from build123d import *

# Parameters (mm, degrees)
SKETCH1_R           = 2.5527
BOSS_EXTRUDE1_DEPTH = 127
SKETCH2_OUTSIDE_W   = 67.612
SKETCH2_OUTSIDE_H   = 65.648
SKETCH2_OUTSIDE_R   = 6.875
CUT_EXTRUDE1_DEPTH  = 25.4
SKETCH3_OUTSIDE_W   = 67.612
SKETCH3_OUTSIDE_H   = 65.648
SKETCH3_OUTSIDE_R   = 6.875
CUT_EXTRUDE2_DEPTH  = 12.7


with BuildPart() as part:
    # Sketch1 → Boss-Extrude1 (new, symmetric)
    with BuildSketch(Plane(origin=(0, 0, 0), x_dir=(0, 0, -1), z_dir=(1, 0, 0))):
        Polygon((3.666174209, -6.35), (7.332348419, 0), (3.666174209, 6.35), (-3.666174209, 6.35), (-7.332348419, 0), (-3.666174209, -6.35), align=None)
        Circle(SKETCH1_R, mode=Mode.SUBTRACT)
    extrude(amount=BOSS_EXTRUDE1_DEPTH, both=True)

    # Sketch2 outside → Cut-Extrude1 (cut)
    with BuildSketch(Plane.ZY.offset(127)):
        Rectangle(SKETCH2_OUTSIDE_W, SKETCH2_OUTSIDE_H)
        Circle(SKETCH2_OUTSIDE_R, mode=Mode.SUBTRACT)
    extrude(amount=-CUT_EXTRUDE1_DEPTH, mode=Mode.SUBTRACT)

    # Sketch3 outside → Cut-Extrude2 (cut)
    with BuildSketch(Plane(origin=(127, 0, 0), x_dir=(0, 0, -1), z_dir=(1, 0, 0))):
        Rectangle(SKETCH3_OUTSIDE_W, SKETCH3_OUTSIDE_H)
        Circle(SKETCH3_OUTSIDE_R, mode=Mode.SUBTRACT)
    extrude(amount=-CUT_EXTRUDE2_DEPTH, mode=Mode.SUBTRACT)


solid = part.part
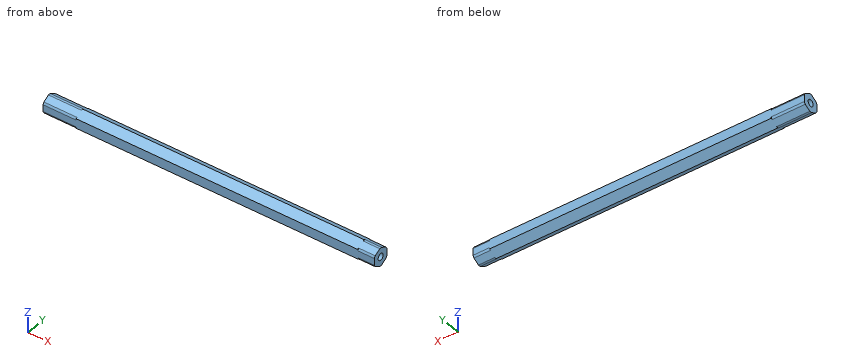
Build history of the part. All positions in model axes, mm. Round coordinates to 2 decimals unless told otherwise and drop trailing zeros. Write each loop counter-clockwise with the first axis right and the second up, starting at its lowest first coordinate (ties: lowest second). Pieces come first, ordered by that corner, then holes. Notation, with made-up numbers: M -3.75,6.5 L 11.25,6.5 A18 ccw 11.25,40.5 Z; hole C -13,-17 d1. An arc over 180 degrees is marked long. Answer as a JSON object with one key per item and string values. Group by question number.
(1) Drill centre lines: L1, parallel to Y at x = 0.5, z = 0.25; L2, parallel to Y at x = 74, z = 0; L3, parallel to Z at x = -50, y = 1.25. Where is each one in solid material? Low to high.
(2) Flat gauge pins, fed straight in: pin 1 (4 mm diameter, centred on y = 0, z = 0, fed in from +X); pin 2 (2 mm diameter, centred on x = 41, y = 3, fed in from +Z). Where does each tip first touch, or does it go through?
(3) Cut at A-A (z = 0). Give the cut face in (x, y).
(4) Cut at B-B (x = -75). Give the cut face in (y, z), and give its area (3 significant figures).
Responses:
{
 "1": {"L1": "y = -6.35 to -2.54, 2.54 to 6.35", "L2": "y = -6.35 to -2.55, 2.55 to 6.35", "L3": "z = -6.61 to -2.23, 2.23 to 6.61"},
 "2": {"pin 1": "passes through", "pin 2": "stops at z = 6.18"},
 "3": {"outline": "M -127,-6.35 L 127,-6.35 L 127,-2.55 L -127,-2.55 Z; M -127,2.55 L 127,2.55 L 127,6.35 L -127,6.35 Z"},
 "4": {"outline": "M -6.35,-3.67 L 0,-7.33 L 6.35,-3.67 L 6.35,3.67 L 0,7.33 L -6.35,3.67 Z; hole C 0,0 d5.11", "area": "119 mm2"}
}
